Check sheet for the modelled part. Datum: model origin and axes. Units: mm. A direction names the side the tool comes from. Round coordinates to 2 decimals unless told otherwise and drop trailing zeros. Loops run counter-clockwise (first coordinate to the right, second up) from the corner with the lowest first, then second, coordinate; pieces in that order, holes last. Notation, with made-up numbers: (31.5, 65) -> (49.5, 65) arc R16 cw to (49.5, 78) -> close; hole circle Ø3 at (18.5, 9). An arc over 180 degrees is marked (long way). Use one line per item in the form item = value. Start each with the question number.
(1) Draft check along X on faces 1 (the flat face through (-47, 23, 25)), 2 (the flat face through (1, 16, 12.5)), 3 (the flat face through (47.87, 15.78, 43.77)). Enter one of: released by +X, released by -X, zero draft, split by the parting line, or undercut.
(2) Sectioned sample at D-D (x = -17). Record the cut outline in (y, z).
(3) Material ranges on probe 1 along Y at (x, z) = (45, 37); probe 2 along Y at (x, z) = (-20.75, 52.25); probe 3 along X at (y, z) = (18, 19) (3 decimals), recorded low to high. Write a range as [from, to].
(4) Set-up check for faces 4 (the flat face through (22, 16, 17.5)), 5 (the cylindrical face through (47.265, 25.713, 18.838)), 6 (the cylindrical face through (-41, 25, 34)): record each of +Z, -Z, +X, -X, +Y, -Y from which the full face is reachable in a straight line by a thin tool's end or side.
(5) Sectioned sample at B-B (z = 39). Record the cut outline in (x, y), and give its area (3 significant figures).
(6) Sectioned sample at C-C (z = 21). State how many separate pieces and enclosed holes the cut face has, and give its area (3 significant figures).
(7) Sectioned sample at A-A (x = 20.75). Record the cut outline in (y, z), and give its area (4 significant figures).
(8) Go/stop test with flat-tipped pins: pin 1 (5 mm diameter, centred on x = 63, y = 25, fed in from +Z); pin 2 (3 mm diameter, centred on x = 20.75, y = 26.25, fed in from +Z); pin 3 (10 mm diameter, centred on x = -52.5, y = 28.5, fed in from +Z); pin 4 (2.5 mm diameter, centred on x = 46, y = 25, fed in from +Z). Record where each tip stops, or that it passes through.
from build123d import *

# Parameters (mm, degrees)
BOSS_EXTRUDE1_DEPTH = 32
FILLET16_R          = 10
FILLET18_R          = 10
FILLET22_R          = 3
FILLET23_R          = 3
FILLET30_R          = 3
FILLET31_R          = 3
FILLET34_R          = 10
FILLET35_R          = 5
SKETCH10_R          = 169.610850048
CUT_EXTRUDE6_DEPTH  = 100.305164141
FILLET37_R          = 10
FILLET38_R          = 20
FILLET39_R          = 10
FILLET40_R          = 20
SKETCH12_W          = 10
SKETCH12_H          = 29.166193857
CUT_EXTRUDE8_DEPTH  = 106.854927259
SKETCH9_R           = 1.75
CUT_EXTRUDE9_DEPTH  = 12.5
FILLET41_R          = 10
FILLET42_R          = 5
SKETCH13_R          = 2.375
CUT_EXTRUDE10_DEPTH = 100.305164141
SKETCH13_3_R        = 4
CUT_EXTRUDE11_DEPTH = 35
FILLET44_R          = 5
FILLET45_R          = 5
BOSS_EXTRUDE2_DEPTH = 32


with BuildPart() as part:
    # Sketch1 → Boss-Extrude1 (new body)
    with BuildSketch(Plane(origin=(0, 0, 0), x_dir=(1, 0, 0), z_dir=(0, 1, 0))):
        with BuildLine():
            Line((22.5, -60), (81.125, -22.5))
            Line((81.125, -22.5), (81.125, 0))
            Line((81.125, 0), (75.125, 0))
            ThreePointArc((75.125, 0), (62.625, -12.5), (50.125, 0))
            Line((50.125, 0), (44.125, 0))
            Line((44.125, 0), (44.125, -12.5))
            Line((44.125, -12.5), (0, -12.5))
            Line((0, -12.5), (0, -60))
            Line((0, -60), (22.5, -60))
        make_face()
        Polygon((26.225, -47.5), (5, -47.5), (5, -17.5), (39.125, -17.5), (39.125, -38.880846325), align=None, mode=Mode.SUBTRACT)
    boss_extrude1 = extrude(amount=BOSS_EXTRUDE1_DEPTH)

    # Mirror1: Boss-Extrude1 across plane
    add(boss_extrude1.mirror(Plane(origin=(0, 32, 0), x_dir=(0, 0, 1), z_dir=(-1, 0, 0))))

    # Fillet16
    fillet16_edges = [part.edges().sort_by_distance(p)[0] for p in [
        (5, 16, 17.5),
    ]]
    fillet(fillet16_edges, radius=FILLET16_R)

    # Fillet18
    fillet18_edges = [part.edges().sort_by_distance(p)[0] for p in [
        (-5, 16, 17.5),
    ]]
    fillet(fillet18_edges, radius=FILLET18_R)

    # Fillet22
    fillet22_edges = [part.edges().sort_by_distance(p)[0] for p in [
        (44.125, 16, 12.5),
    ]]
    fillet(fillet22_edges, radius=FILLET22_R)

    # Fillet23
    fillet23_edges = [part.edges().sort_by_distance(p)[0] for p in [
        (-44.125, 16, 12.5),
    ]]
    fillet(fillet23_edges, radius=FILLET23_R)

    # Fillet30
    fillet30_edges = [part.edges().sort_by_distance(p)[0] for p in [
        (81.125, 16, 22.5),
    ]]
    fillet(fillet30_edges, radius=FILLET30_R)

    # Fillet31
    fillet31_edges = [part.edges().sort_by_distance(p)[0] for p in [
        (-81.125, 16, 22.5),
    ]]
    fillet(fillet31_edges, radius=FILLET31_R)

    # Fillet34
    fillet34_edges = [part.edges().sort_by_distance(p)[0] for p in [
        (5, 16, 47.5),
    ]]
    fillet(fillet34_edges, radius=FILLET34_R)

    # Fillet35
    fillet35_edges = [part.edges().sort_by_distance(p)[0] for p in [
        (-26.225, 16, 47.5),
    ]]
    fillet(fillet35_edges, radius=FILLET35_R)

    # Sketch10 → Cut-Extrude6 (cut, through all)
    with BuildSketch(Plane(origin=(0, 0, 12.5), x_dir=(-1, 0, 0), z_dir=(0, 0, -1))):
        Circle(SKETCH10_R)
    extrude(amount=CUT_EXTRUDE6_DEPTH, mode=Mode.SUBTRACT)

    # Fillet37
    fillet37_edges = [part.edges().sort_by_distance(p)[0] for p in [
        (39.125, 16, 17.5),
    ]]
    fillet(fillet37_edges, radius=FILLET37_R)

    # Fillet38
    fillet38_edges = [part.edges().sort_by_distance(p)[0] for p in [
        (39.125, 16, 38.880846325),
    ]]
    fillet(fillet38_edges, radius=FILLET38_R)

    # Fillet39
    fillet39_edges = [part.edges().sort_by_distance(p)[0] for p in [
        (-39.125, 16, 17.5),
    ]]
    fillet(fillet39_edges, radius=FILLET39_R)

    # Fillet40
    fillet40_edges = [part.edges().sort_by_distance(p)[0] for p in [
        (-39.125, 16, 38.880846325),
    ]]
    fillet(fillet40_edges, radius=FILLET40_R)

    # Sketch12 → Cut-Extrude8 (cut, through all)
    with BuildSketch(Plane(origin=(0, 0, 0), x_dir=(-1, 0, 0), z_dir=(0, -1, 0))):
        with Locations((-76.125, -27.083096929)):
            Rectangle(SKETCH12_W, SKETCH12_H)
    cut_extrude8 = extrude(amount=-CUT_EXTRUDE8_DEPTH, mode=Mode.SUBTRACT)

    # Sketch9 → Cut-Extrude9 (cut)
    with BuildSketch(Plane.XY.offset(60)):
        with Locations((-20.75, 5.75)):
            Circle(SKETCH9_R)
        with Locations((-20.75, 26.25)):
            Circle(SKETCH9_R)
    cut_extrude9 = extrude(amount=-CUT_EXTRUDE9_DEPTH, mode=Mode.SUBTRACT)

    # Fillet41
    fillet41_edges = [part.edges().sort_by_distance(p)[0] for p in [
        (-5, 16, 47.5),
    ]]
    fillet(fillet41_edges, radius=FILLET41_R)

    # Fillet42
    fillet42_edges = [part.edges().sort_by_distance(p)[0] for p in [
        (26.225, 16, 47.5),
    ]]
    fillet(fillet42_edges, radius=FILLET42_R)

    # Mirror5: Cut-Extrude9 across plane
    add(cut_extrude9.mirror(Plane(origin=(0, 0, 0), x_dir=(0, 0, 1), z_dir=(1, 0, 0))), mode=Mode.SUBTRACT)

    # Sketch13 → Cut-Extrude10 (cut, symmetric)
    with BuildSketch(Plane.XY.offset(60)):
        with Locations((45, 7.15)):
            Circle(SKETCH13_R)
        with Locations((45, 25)):
            Circle(SKETCH13_R)
        with Locations((63, 25)):
            Circle(SKETCH13_R)
        with Locations((63, 7)):
            Circle(SKETCH13_R)
    cut_extrude10 = extrude(amount=CUT_EXTRUDE10_DEPTH, both=True, mode=Mode.SUBTRACT)

    # Sketch13<3> → Cut-Extrude11 (cut)
    with BuildSketch(Plane.XY.offset(60)):
        with Locations((45, 7.15)):
            Circle(SKETCH13_3_R)
        with Locations((45, 25)):
            Circle(SKETCH13_3_R)
        with Locations((63, 25)):
            Circle(SKETCH13_3_R)
        with Locations((63, 7)):
            Circle(SKETCH13_3_R)
    cut_extrude11 = extrude(amount=-CUT_EXTRUDE11_DEPTH, mode=Mode.SUBTRACT)

    # Mirror6: Cut-Extrude10, Cut-Extrude11 across plane
    add(cut_extrude10.mirror(Plane(origin=(0, 0, 0), x_dir=(0, 0, 1), z_dir=(1, 0, 0))), mode=Mode.SUBTRACT)
    add(cut_extrude11.mirror(Plane(origin=(0, 0, 0), x_dir=(0, 0, 1), z_dir=(1, 0, 0))), mode=Mode.SUBTRACT)

    # Fillet44
    fillet44_edges = [part.edges().sort_by_distance(p)[0] for p in [
        (71.125, 16, 28.896588486),
        (71.125, 32, 20.698294243),
        (71.125, 0, 20.698294243),
    ]]
    fillet(fillet44_edges, radius=FILLET44_R)

    # Mirror7: Cut-Extrude8 across plane
    add(cut_extrude8.mirror(Plane(origin=(0, 0, 0), x_dir=(0, 0, 1), z_dir=(1, 0, 0))), mode=Mode.SUBTRACT)

    # Fillet45
    fillet45_edges = [part.edges().sort_by_distance(p)[0] for p in [
        (-71.125, 16, 28.896588486),
        (-71.125, 32, 20.698294243),
        (-71.125, 0, 20.698294243),
    ]]
    fillet(fillet45_edges, radius=FILLET45_R)

    # Sketch14 → Boss-Extrude2 (add)
    with BuildSketch(Plane.XZ):
        Polygon((-27.5, 56.801705757), (-22.5, 60), (-27.5, 60), align=None)
    boss_extrude2 = extrude(amount=-BOSS_EXTRUDE2_DEPTH)

    # Mirror8: Boss-Extrude2 across plane
    add(boss_extrude2.mirror(Plane(origin=(0, 0, 0), x_dir=(0, 0, 1), z_dir=(1, 0, 0))))


solid = part.part
Checks:
q1.face_1 = undercut
q1.face_2 = zero draft
q1.face_3 = released by +X
q2.outline = (0, 12.5) -> (32, 12.5) -> (32, 17.5) -> (0, 17.5) -> close; (0, 47.5) -> (32, 47.5) -> (32, 60) -> (0, 60) -> close
q3.probe_1 = [0, 3.15], [11.15, 21], [29, 32]
q3.probe_2 = [0, 4], [7.5, 24.5], [28, 32]
q3.probe_3 = [-71.125, -34.393], [-9.732, 9.732], [34.393, 71.125]
q4.face_4 = +Y, -Y
q4.face_5 = +Z, -Z
q4.face_6 = +Z
q5.outline = (-55.33, 0) -> (-35.95, 0) -> (-35.95, 32) -> (-55.33, 32) -> close; (-5.11, 0) -> (5.11, 0) -> (5.11, 32) -> (-5.11, 32) -> close; (35.95, 0) -> (55.33, 0) -> (55.33, 32) -> (35.95, 32) -> close; hole circle Ø8 at (-45, 7.15); hole circle Ø8 at (-45, 25); hole circle Ø8 at (45, 7.15); hole circle Ø8 at (45, 25)
q5.area = 1,370 mm2
q6.separate_pieces = 3
q6.enclosed_holes = 8
q6.area = 2,510 mm2
q7.outline = (0, 12.5) -> (32, 12.5) -> (32, 17.5) -> (0, 17.5) -> close; (0, 47.5) -> (4, 47.5) -> (4, 60) -> (0, 60) -> close; (7.5, 47.5) -> (24.5, 47.5) -> (24.5, 60) -> (7.5, 60) -> close; (28, 47.5) -> (32, 47.5) -> (32, 60) -> (28, 60) -> close
q7.area = 472.5 mm2
q8.pin_1 = 25
q8.pin_2 = 17.5
q8.pin_3 = 44.01
q8.pin_4 = through
